CAD build for the part. Positions are in the model's coordinates, mm. A direction names the side the tool comes from. Round coordinates to 2 decimals unless told otherwise and drop trailing zeros. Write each loop counter-clockwise with the first axis right and the second up, starting at its lowest first coordinate (ties: lowest second). Pieces come first, ordered by that corner, then holes. Notation, with made-up numbers: (45, -29) - (49, -29) arc R21 cw to (49, -3) - close; hole circle Ø8 at (83.25, -20). An arc over 180 degrees is marked (long way). Answer in a Markdown table with one row per item.
```python
from build123d import *

# Parameters (mm, degrees)
SKETCH1_W           = 12.25
SKETCH1_H           = 10.5
BOSS_EXTRUDE1_DEPTH = 16.5
CUT_EXTRUDE1_DEPTH  = 15
FILLET1_R           = 0.5
SKETCH8_W           = 7.057916012
SKETCH8_H           = 2.856354625
BOSS_EXTRUDE3_DEPTH = 0.2
SKETCH4_W           = 7.057916012
SKETCH4_H           = 2.856354625
BOSS_EXTRUDE4_DEPTH = 0.2


with BuildPart() as part:
    # Sketch1 → Boss-Extrude1 (new body)
    with BuildSketch(Plane.XY):
        with Locations((6.125, 5.25)):
            Rectangle(SKETCH1_W, SKETCH1_H)
    extrude(amount=-BOSS_EXTRUDE1_DEPTH)

    # Sketch3 → Cut-Extrude1 (cut)
    with BuildSketch(Plane.XY):
        with BuildLine():
            Line((1.5, 6.167157288), (1.5, 1.7))
            ThreePointArc((1.5, 1.7), (1.558578644, 1.558578644), (1.7, 1.5))
            Line((1.7, 1.5), (10.55, 1.5))
            ThreePointArc((10.55, 1.5), (10.691421356, 1.558578644), (10.75, 1.7))
            Line((10.75, 1.7), (10.75, 6.167157288))
            ThreePointArc((10.75, 6.167157288), (10.734775907, 6.243693974), (10.691421356, 6.308578644))
            Line((10.691421356, 6.308578644), (8.058578644, 8.941421356))
            ThreePointArc((8.058578644, 8.941421356), (7.993693974, 8.984775907), (7.917157288, 9))
            Line((7.917157288, 9), (4.332842712, 9))
            ThreePointArc((4.332842712, 9), (4.256306026, 8.984775907), (4.191421356, 8.941421356))
            Line((4.191421356, 8.941421356), (1.558578644, 6.308578644))
            ThreePointArc((1.558578644, 6.308578644), (1.515224093, 6.243693974), (1.5, 6.167157288))
        make_face()
        with BuildLine():
            ThreePointArc((3.825, 6), (3.683578644, 5.941421356), (3.625, 5.8))
            Line((3.625, 5.8), (3.625, 3.7))
            ThreePointArc((3.625, 3.7), (3.683578644, 3.558578644), (3.825, 3.5))
            Line((3.825, 3.5), (8.425, 3.5))
            ThreePointArc((8.425, 3.5), (8.566421356, 3.558578644), (8.625, 3.7))
            Line((8.625, 3.7), (8.625, 5.8))
            ThreePointArc((8.625, 5.8), (8.566421356, 5.941421356), (8.425, 6))
            Line((8.425, 6), (3.825, 6))
        make_face(mode=Mode.SUBTRACT)
    extrude(amount=-CUT_EXTRUDE1_DEPTH, mode=Mode.SUBTRACT)

    # Fillet1
    fillet1_edges = [part.edges().sort_by_distance(p)[0] for p in [
        (12.25, 5.25, -16.5),
        (6.125, 10.5, -16.5),
        (8.625, 4.75, -15),
        (8.566421356, 5.941421356, -15),
        (6.125, 6, -15),
        (3.683578644, 5.941421356, -15),
        (3.625, 4.75, -15),
        (3.683578644, 3.558578644, -15),
        (6.125, 3.5, -15),
        (8.566421356, 3.558578644, -15),
        (0, 5.25, -16.5),
        (6.125, 10.5, 0),
        (12.25, 5.25, 0),
        (6.125, 0, 0),
        (0, 5.25, 0),
        (0, 10.5, -8.25),
        (12.25, 10.5, -8.25),
        (12.25, 0, -8.25),
        (0, 0, -8.25),
    ]]
    fillet(fillet1_edges, radius=FILLET1_R)

    # Sketch8 → Boss-Extrude3 (add)
    with BuildSketch(Plane(origin=(1.5, 0, 0), x_dir=(0, 0, -1), z_dir=(1, 0, 0))):
        with Locations((3.528958006, 4.738979976)):
            Rectangle(SKETCH8_W, SKETCH8_H)
    extrude(amount=BOSS_EXTRUDE3_DEPTH)

    # Sketch4 → Boss-Extrude4 (add)
    with BuildSketch(Plane.ZY.offset(-10.75)):
        with Locations((-3.528958006, 4.738979976)):
            Rectangle(SKETCH4_W, SKETCH4_H)
    extrude(amount=BOSS_EXTRUDE4_DEPTH)


solid = part.part
```
Q1. Saw through at D-D on x = 7.5. List the corners of the cut face in (y, z).
Computed:
| item | result |
|---|---|
| outline | (0, -16.5) - (10, -16.5) arc R0.5 ccw to (10.5, -16) - (10.5, -0.5) arc R0.5 ccw to (10, 0) - (9, 0) - (9, -15) - (6.5, -15) arc R0.5 cw to (6, -14.5) - (6, 0) - (3.5, 0) - (3.5, -14.5) arc R0.5 cw to (3, -15) - (1.5, -15) - (1.5, 0) - (0.5, 0) arc R0.5 ccw to (0, -0.5) - close |
Q2. Drill centre lines: line 1 (X direction, y = 4.5, z = -11.25) (3 decimals); line 2 (Y direction, x = 5.75, z = -1); line 3 (X direction, y = 2.75, z = -14.75). Where is each one in solid material? Low to high.
Computed:
| item | result |
|---|---|
| line 1 | x = 0 to 1.5, 3.625 to 8.625, 10.75 to 12.25 |
| line 2 | y = 0 to 1.5, 3.5 to 6, 9 to 10.5 |
| line 3 | x = 0 to 1.5, 10.75 to 12.25 |
Q3. Pull direction Y, two halves, no side cores. Call faces 4 (the flat face through (12.25, 5, -8)), 5 (the flat face through (10.75, 3, -9)), 6 (the flat face through (6, 0, -8)): released by +Y, released by -Y, zero draft, split by the parting line, or undercut.
Computed:
| item | result |
|---|---|
| face 4 | zero draft |
| face 5 | undercut |
| face 6 | released by -Y |
Q4. Saw through at B-B on x = 10.25. List the corners of the cut face in (y, z), then the cut area to 3 significant figures.
Computed:
| item | result |
|---|---|
| outline | (0, -16.5) - (10, -16.5) arc R0.5 ccw to (10.5, -16) - (10.5, -0.5) arc R0.5 ccw to (10, 0) - (6.75, 0) - (6.75, -15) - (1.5, -15) - (1.5, 0) - (0.5, 0) arc R0.5 ccw to (0, -0.5) - close |
| area | 94.3 mm2 |
Q5. Saw through at A-A on z = -12. List the corners of the cut face in (x, y) (3 decimals).
Computed:
| item | result |
|---|---|
| outline | (0, 0.5) arc R0.5 ccw to (0.5, 0) - (11.75, 0) arc R0.5 ccw to (12.25, 0.5) - (12.25, 10) arc R0.5 ccw to (11.75, 10.5) - (0.5, 10.5) arc R0.5 ccw to (0, 10) - close; (3.625, 3.7) arc R0.2 ccw to (3.825, 3.5) - (8.425, 3.5) arc R0.2 ccw to (8.625, 3.7) - (8.625, 5.8) arc R0.2 ccw to (8.425, 6) - (3.825, 6) arc R0.2 ccw to (3.625, 5.8) - close; hole (1.5, 1.7) arc R0.2 ccw to (1.7, 1.5) - (10.55, 1.5) arc R0.2 ccw to (10.75, 1.7) - (10.75, 6.167) arc R0.2 ccw to (10.691, 6.309) - (8.059, 8.941) arc R0.2 ccw to (7.917, 9) - (4.333, 9) arc R0.2 ccw to (4.191, 8.941) - (1.559, 6.309) arc R0.2 ccw to (1.5, 6.167) - close |
Q6. Saw through at C-C on y = 5.5. List the corners of the cut face in (x, z) (3 decimals).
Computed:
| item | result |
|---|---|
| outline | (0, -16) arc R0.5 ccw to (0.5, -16.5) - (11.75, -16.5) arc R0.5 ccw to (12.25, -16) - (12.25, -0.5) arc R0.5 ccw to (11.75, 0) - (10.55, 0) - (10.55, -7.058) - (10.75, -7.058) - (10.75, -15) - (9.125, -15) arc R0.5 cw to (8.625, -14.5) - (8.625, 0) - (3.625, 0) - (3.625, -14.5) arc R0.5 cw to (3.125, -15) - (1.5, -15) - (1.5, -7.058) - (1.7, -7.058) - (1.7, 0) - (0.5, 0) arc R0.5 ccw to (0, -0.5) - close |
Q7. 3-axis set-ups, long thin cutter, end or side, ignore diameter. For faces 1 (the flat face through (1.5, 3, -9)), 2 (the flat face through (3.625, 5, -7)), 3 (the flat face through (6, 10.5, -8)): which of +Z, -Z, +X, -X, +Y, -Y reach the whole face in a straight line?
Computed:
| item | result |
|---|---|
| face 1 | none |
| face 2 | +Z |
| face 3 | +Z, -Z, +X, -X, +Y |
